```python
from build123d import *

# Parameters (mm, degrees)
F0_R     = 25.4
F1_DEPTH = 12.7


with BuildPart() as f1:
    # F0 (on Top) → F1 (new body, symmetric)
    with BuildSketch(Plane.XY):
        Circle(F0_R)
        with BuildLine():
            ThreePointArc((-12.7, -6.35), (-8.209872, -8.209872), (-6.35, -12.7))
            Line((-6.35, -12.7), (-6.35, -18.494382))
            ThreePointArc((-6.35, -18.494382), (-7.241618, -20.133529), (-9.102152, -20.275637))
            ThreePointArc((-9.102152, -20.275637), (-15.715448, -15.715448), (-20.275637, -9.102152))
            ThreePointArc((-20.275637, -9.102152), (-20.133529, -7.241617), (-18.494382, -6.35))
            Line((-18.494382, -6.35), (-12.7, -6.35))
        make_face(mode=Mode.SUBTRACT)
        with BuildLine():
            ThreePointArc((0, 6.35), (4.490128, 4.490128), (6.35, 0))
            ThreePointArc((6.35, 0), (4.490128, -4.490128), (0, -6.35))
            ThreePointArc((0, -6.35), (-4.490128, -4.490128), (-6.35, 0))
            ThreePointArc((-6.35, 0), (-4.490128, 4.490128), (0, 6.35))
        make_face(mode=Mode.SUBTRACT)
        with BuildLine():
            ThreePointArc((6.35, -12.7), (8.209872, -8.209872), (12.7, -6.35))
            Line((12.7, -6.35), (18.494382, -6.35))
            ThreePointArc((18.494382, -6.35), (20.133529, -7.241618), (20.275637, -9.102152))
            ThreePointArc((20.275637, -9.102152), (15.715448, -15.715448), (9.102152, -20.275637))
            ThreePointArc((9.102152, -20.275637), (7.241617, -20.133529), (6.35, -18.494382))
            Line((6.35, -18.494382), (6.35, -12.7))
        make_face(mode=Mode.SUBTRACT)
        with BuildLine():
            ThreePointArc((-20.275637, 9.102152), (-15.715448, 15.715448), (-9.102152, 20.275637))
            ThreePointArc((-9.102152, 20.275637), (-7.241618, 20.133529), (-6.35, 18.494382))
            Line((-6.35, 18.494382), (-6.35, 12.7))
            ThreePointArc((-6.35, 12.7), (-8.209872, 8.209872), (-12.7, 6.35))
            Line((-12.7, 6.35), (-18.494382, 6.35))
            ThreePointArc((-18.494382, 6.35), (-20.133529, 7.241618), (-20.275637, 9.102152))
        make_face(mode=Mode.SUBTRACT)
        with BuildLine():
            ThreePointArc((12.7, 6.35), (8.209872, 8.209872), (6.35, 12.7))
            Line((6.35, 12.7), (6.35, 18.494382))
            ThreePointArc((6.35, 18.494382), (7.241618, 20.133529), (9.102152, 20.275637))
            ThreePointArc((9.102152, 20.275637), (15.715448, 15.715448), (20.275637, 9.102152))
            ThreePointArc((20.275637, 9.102152), (20.133529, 7.241618), (18.494382, 6.35))
            Line((18.494382, 6.35), (12.7, 6.35))
        make_face(mode=Mode.SUBTRACT)
    extrude(amount=F1_DEPTH, both=True)


solid = f1.part
```
Here's how the part is built. I have some questions about the finished solid (model axes, mm). Give positions to 0.01 mm unless a question says otherwise; leave off trailing zeros. Write each loop counter-clockwise with the first axis right and the second up, starting at its lowest first coordinate (ties: lowest second). Pieces come first, ordered by that corner, then holes. Notation, with made-up numbers: (86.25, 82) -> (141.25, 82) arc R21 ccw to (141.25, 96) -> close; hole circle Ø5 at (-11.75, 57). An arc over 180 degrees is marked (long way). Use one line per item in the form item = value.
1) Suppose I cut it at C-C (z = -4.75). Give the number of separate pieces and of enclosed holes in the cut face, and give its area (3 significant figures).
Verdict:
separate_pieces = 1
enclosed_holes = 5
area = 1,350 mm2
2) Suppose I cut it at B-B (y = 2.5). Please give me the cut outline in (x, z).
Verdict:
outline = (-25.28, -12.7) -> (-5.84, -12.7) -> (-5.84, 12.7) -> (-25.28, 12.7) -> close; (5.84, -12.7) -> (25.28, -12.7) -> (25.28, 12.7) -> (5.84, 12.7) -> close
3) I'm going to push flat-ended pins straight in: pin 1 (3 mm diameter, centred on x = -4.5, y = 1, fed in from +Z); pin 2 (3 mm diameter, centred on x = -14.5, z = -4.5, fed in from -Y); pin 3 (10 mm diameter, centred on x = 1.5, z = 3.5, fed in from +Y); pin 4 (1.5 mm diameter, centred on y = 14.5, z = 6, fed in from +X). Where does each tip first touch, or does it pass through?
Verdict:
pin_1 = through
pin_2 = -21.82
pin_3 = 25.4
pin_4 = 21.36
4) We'd pull the mould along X, two halves only. Please class faces 1 (the face through (-7.265, 20.148, 0.178)), 2 (the face through (5, -5, -12.7)): +X half, -X half, draft (parallel to the pull), parting line (faces both ways), or undercut.
Verdict:
face_1 = undercut
face_2 = draft
5) Suppose I cut it at A-A (x = 2). Please give me the cut outline in (y, z), and give its area (3 significant figures).
Verdict:
outline = (-25.32, -12.7) -> (-6.03, -12.7) -> (-6.03, 12.7) -> (-25.32, 12.7) -> close; (6.03, -12.7) -> (25.32, -12.7) -> (25.32, 12.7) -> (6.03, 12.7) -> close
area = 980 mm2
6) If I drill on L1, parallel to Y at x = -19, z = 10.25; L2, parallel to X at y = 10, z = 6.75; L3, parallel to X at y = 18, z = -10, over which ranges is the centre line in solid material (lowest first)? Write a range as [from, to].
Verdict:
L1 = [-16.86, -11.53], [-6.42, 6.42], [11.53, 16.86]
L2 = [-23.35, -19.85], [-6.95, 6.95], [19.85, 23.35]
L3 = [-17.92, -13.04], [-6.35, 6.35], [13.04, 17.92]
7) Suppose I cut it at D-D (y = 21.5). Please give me the cut outline in (x, z), and give its area (3 significant figures).
Verdict:
outline = (-13.52, -12.7) -> (13.52, -12.7) -> (13.52, 12.7) -> (-13.52, 12.7) -> close
area = 687 mm2
